Autodesk Inventor part; units mm, degrees
ref_plane "YZ Plane" through (0, 0, 0) normal (1, 0, 0) x (0, 1, 0)
ref_plane "XZ Plane" through (0, 0, 0) normal (0, 1, 0) x (-1, 0, 0)
ref_plane "XY Plane" through (0, 0, 0) normal (0, 0, 1) x (1, 0, 0)
sketch "Sketch1" plane through (0, 0, 0) normal (0, 0, 1) x (1, 0, 0)
  line L0 (0, 0) -> (34, 0)
  line L1 (34, 0) -> (34, 74)
  line L2 (34, 74) -> (0, 74)
  line L3 (0, 74) -> (0, 0)
  line L4 (33, 73) -> (1, 73)
  line L5 (1, 73) -> (1, 1)
  line L6 (1, 1) -> (33, 1)
  line L7 (33, 1) -> (33, 73)
  dimension "d0" = 34
  dimension "d1" = 74
  dimension "d2" = 1
  dimension "d3" = 1
  dimension "d4" = 1
  dimension "d5" = 1
extrude "Extrusion1" add sketch "Sketch1" along normal blind 1.5 contours L3 L2 L1 L0 | L7 L6 L5 L4
extrude "Extrusion2" add sketch "Sketch1" along normal blind 20
sketch "Sketch2" plane through (0, 0, 0) normal (0, 0, -1) x (-1, 0, 0)
  circle A0 centre (-32, 2) radius 1
  circle A1 centre (-2, 72) radius 1
  line L0 (0, 74) -> (0, 0)
  line L1 (-34, 74) -> (0, 74)
  line L2 (0, 0) -> (-34, 0)
  line L3 (-34, 0) -> (-34, 74)
  dimension "d10" = 2
  dimension "d11" = 2
  dimension "d12" = 2
  dimension "d13" = 2
  dimension "d14" = 2
  dimension "d15" = 2
extrude "Extrusion3" cut sketch "Sketch2" against normal through all contours A0 | A1
sketch "Sketch3" plane through (0, 0, 20) normal (0, 0, 1) x (1, 0, 0)
  line L0 (34, 74) -> (0, 74)
  line L1 (34, 0) -> (34, 74)
  line L2 (0, 74) -> (34, 74)
  line L3 (34, 74) -> (34, 69)
  line L4 (34, 69) -> (0, 69)
  line L5 (0, 69) -> (0, 74)
  line L6 (34, 0) -> (29, 0)
  line L7 (29, 0) -> (29, 5)
  line L8 (29, 5) -> (34, 5)
  line L9 (34, 5) -> (34, 0)
  point P0 (0, 0)
  dimension "d20" = 5
  dimension "d21" = 5
  dimension "d22" = 5
extrude "Extrusion4" cut sketch "Sketch3" against normal blind 8
chamfer "Chamfer1" distance 1.5 angle 45 2 edges at (3, 72, 0) (33, 2, 0)
properties part number "brainholder"
Geometry check sheet. Reference: the model listing, model coordinates, mm. A direction names the side the tool comes from. Give positions to 0.01 mm unless a question says otherwise; leave off trailing zeros. Order: outer loops, then holes, each group sorted by start corner. A loop starts at its lowest first (then second) coordinate and runs counter-clockwise, first axis right, second up.
1) Cross-section at D-D (x = 21). Record the boundary of the cut face in (y, z), then the cut area to 3 significant figures.
Results are:
outline: (0, 0) - (74, 0) - (74, 12) - (73, 12) - (73, 1.5) - (1, 1.5) - (1, 20) - (0, 20) - close
area: 140 mm2
2) Cross-section at A-A (z = 13.5). Record the boundary of the cut face in (x, y), then the cut area to 3 significant figures.
Results are:
outline: (0, 0) - (29, 0) - (29, 1) - (1, 1) - (1, 69) - (0, 69) - close; (33, 5) - (34, 5) - (34, 69) - (33, 69) - close
area: 161 mm2
3) Gauge pin test, flat ends, axial feed: pin 1 (0.8 mm diameter, centred on x = 33.5, z = 14, fed in from +Y); pin 2 (0.5 mm diameter, centred on x = 1.5, y = 72.5, fed in from +Z); pin 3 (2 mm diameter, centred on x = 4.5, y = 25, fed in from +Z). Record the tip position at first contact, or that the pin passes through.
Results are:
pin 1: stops at y = 69
pin 2: passes through
pin 3: stops at z = 1.5
4) Cross-section at B-B (z = 8.25). Record the boundary of the cut face in (x, y).
Results are:
outline: (0, 0) - (34, 0) - (34, 74) - (0, 74) - close; hole (1, 1) - (33, 1) - (33, 73) - (1, 73) - close
5) Material ranges on probe 1 along Y at (x, z) = (15, 6); probe 2 along X at (y, z) = (12, 7.5); probe 3 along Z at (x, y) = (5, 25.5), recorded low to high.
Results are:
probe 1: y = 0 to 1, 73 to 74
probe 2: x = 0 to 1, 33 to 34
probe 3: z = 0 to 1.5
6) Draft check along X on faces 6 (the flat face through (17, 1, 11)), 7 (the flat face through (17, 0, 10)), 8 (the flat face through (34, 36, 10)). Enter one of: released by +X, released by -X, zero draft, split by the parting line, or undercut.
Results are:
face 6: undercut
face 7: zero draft
face 8: released by +X
7) Cross-section at C-C (y = 42). Record the boundary of the cut face in (x, z), then the cut area to 3 significant figures.
Results are:
outline: (0, 0) - (34, 0) - (34, 20) - (33, 20) - (33, 1.5) - (1, 1.5) - (1, 20) - (0, 20) - close
area: 88.0 mm2
8) Tool access check on faces 1 (the flat face through (16.9, 73.4, 12)), 2 (the flat face through (33.13, 0.87, 12)), 3 (the flat face through (0.5, 34.7, 20)), 4 (the flat face through (17, 38, 1.5)), 5 (the conical face through (3, 71.23, 1.24)). Record the directions out of +Z, -Z, +X, -X, +Y, -Y that give a thin tool (end or side, any length) a straight path to the whole face; none if there is none.
Results are:
face 1: +Z, +X, -X, +Y
face 2: +Z, +X, -Y
face 3: +Z, +X, -X, +Y, -Y
face 4: +Z
face 5: -Z
